Here's how the part is built. I have some questions about the finished solid (model axes, mm). A direction names the side the tool comes from. Give positions to 0.01 mm unless a question says otherwise; leave off trailing zeros. Write each loop counter-clockwise with the first axis right and the second up, starting at its lowest first coordinate (ties: lowest second). Pieces come first, ordered by that corner, then holes. Notation, with made-up numbers: (-7.75, 36) - (17.25, 36) arc R9 ccw to (17.25, 49) - close; hole circle Ø7 at (7, -1.75). An arc over 180 degrees is marked (long way). Write each question's results on one line, items separated by ' | '. Start each with the question number.
Item 1: Which directions (+Z, -Z, +X, -X, +Y, -Y) give clear straight access to the entire face, cutting with the end or side of a thin tool? Please do faces 5 (the flat face through (-1, -9, 0)), 6 (the flat face through (2, -4, -2.5)), 7 (the cylindrical face through (-1, 0, 0)).
Item 2: We'd pull the mould along Y, two halves only. Please class faces 1 (the cylindrical face through (2, -12, 0)), 2 (the cylindrical face through (0.01, -8.51, -0.13)), 3 (the flat face through (2, -4, 2.5)), 4 (the flat face through (1.15, 1, 0.04)): +Y half, -Y half, draft (parallel to the pull), parting line (faces both ways), or undercut.
Item 3: Suppose I cut it at C-C on y = -0.5. List the corners of the cut face in (x, z) for me, then the cut area to 3 significant figures.
Item 4: Will these pins go through, and if not, where does the flat tip stop? P1, Ø2, axis at x = -0.5, z = 1, coming from the -Y side; P2, Ø2, axis at y = -10, z = -0.5, coming from the -X side; P3, Ø1.5, axis at y = -7.5, z = 0.5, coming from the -X side.
Item 5: Suppose I cut it at B-B on z = -0.7. List the corners of the cut face in (x, y) for me.
Item 6: Please list where these lines run through material, in increasing order: line 1 along Z through (x, y) = (0, -0.5); line 2 along X through (y, z) = (-8.5, -1.8).
Item 7: Suppose I cut it at D-D on x = 1.75. List the corners of the cut face in (y, z) for me, then the cut area to 3 significant figures.
Item 8: Suppose I cut it at A-A on x = 0. List the corners of the cut face in (y, z) for me, then the cut area to 3 significant figures.
```python
from build123d import *

# Parameters (mm, degrees)
SKETCH1_R           = 2.5
SKETCH1_R_2         = 1
BOSS_EXTRUDE1_DEPTH = 1
BOSS_EXTRUDE2_DEPTH = 1.5
SKETCH5_R           = 1
BOSS_EXTRUDE3_DEPTH = 2


with BuildPart() as part:
    # Sketch1 → Boss-Extrude1 (new, symmetric)
    with BuildSketch(Plane(origin=(0, 0, 0), x_dir=(1, 0, 0), z_dir=(0, 1, 0))):
        with Locations(Location((0, 0, 0), (0, 0, 270))):
            Circle(SKETCH1_R)
        with Locations(Location((0, 0, 0), (0, 0, 270))):
            Circle(SKETCH1_R_2, mode=Mode.SUBTRACT)
    extrude(amount=BOSS_EXTRUDE1_DEPTH, both=True)

    # Sketch2 → Boss-Extrude2 (add)
    with BuildSketch(Plane(origin=(2.5, 0, 0), x_dir=(0, 0, -1), z_dir=(1, 0, 0))):
        with BuildLine():
            Line((-2.5, 1), (2.5, 1))
            Line((2.5, 1), (2.5, -9.5))
            ThreePointArc((2.5, -9.5), (0, -12), (-2.5, -9.5))
            Line((-2.5, -9.5), (-2.5, 1))
        make_face()
    extrude(amount=-BOSS_EXTRUDE2_DEPTH)

    # Sketch5 → Boss-Extrude3 (add)
    with BuildSketch(Plane.ZY.offset(-1)):
        with Locations((0, -9.5)):
            Circle(SKETCH5_R)
    extrude(amount=BOSS_EXTRUDE3_DEPTH)


solid = part.part
```
Checked values:
1) face 5: +Z, -Z, -X, -Y | face 6: -Z, +X, -X, +Y, -Y | face 7: +Y
2) face 1: -Y half | face 2: undercut | face 3: draft | face 4: +Y half
3) outline: (1, -2.5) - (2.5, -2.5) - (2.5, 2.5) - (1, 2.5) - (1, 2.29) arc R2.5 ccw (long way) to (1, -2.29) - close; hole circle Ø2 at (0, 0) | area: 19.0 mm^2
4) P1: stops at y = -10.5 | P2: stops at x = -1 | P3: stops at x = 1
5) outline: (-2.4, -1) - (-0.71, -1) - (-0.71, 1) - (-2.4, 1) - close; (-1, -10.21) - (1, -10.21) - (1, -11.9) - (2.5, -11.9) - (2.5, 1) - (0.71, 1) - (0.71, -1) - (1, -1) - (1, -8.79) - (-1, -8.79) - close
6) line 1: z = -2.5 to -1, 1 to 2.5 | line 2: x = 1 to 2.5
7) outline: (-9.5, -2.5) - (1, -2.5) - (1, 2.5) - (-9.5, 2.5) arc R2.5 ccw to start | area: 62.3 mm^2
8) outline: circle Ø2 at (-9.5, 0); (-1, -2.5) - (1, -2.5) - (1, -1) - (-1, -1) - close; (-1, 1) - (1, 1) - (1, 2.5) - (-1, 2.5) - close | area: 9.14 mm^2
